Here's how the part is built. I have some questions about the finished solid (model axes, mm). Face numbers are marked on the shaded views. A direction names the side the tool comes from. Give positions to 0.01 mm unless a question says otherwise; leave off trailing zeros. Write each loop counter-clockwise with the first axis right and the second up, starting at its lowest first coordinate (ties: lowest second). Pieces come first, ordered by that corner, then holes. Notation, with made-up numbers: (42.5, 75) - (95.5, 75) arc R10 cw to (95.5, 88) - close; hole circle Ø2 at (88, -6.75). An arc over 180 degrees is marked (long way). One line per item, written item: value. Start each with the question number.
1) Imagine slicing it at D-D on x = 88. Write out the boundary of the cut face in (y, z), plus the area to 3 significant figures.
2) On a 3-axis mill with a long thin cutter (end or side, diameter ignored), from which of +Z, -Z, +X, -X, +Y, -Y can I reach the whole of each face in a straight line? I mean the marked faces 1 and 2. Say none if no direction works.
3) Imagine slicing it at A-A on x = 49.5. Write out the boundary of the cut face in (y, z), plus the area to 3 significant figures.
4) Imagine slicing it at C-C on y = 43.5. Write out the boundary of the cut face in (x, z), plus the area to 3 significant figures.
5) Imagine slicing it at B-B on z = 32. Write out the boundary of the cut face in (x, y).
6) I'm going to push flat-ended pins straight in: P1, Ø1, axis at x = 88.5, y = 43.5, coming from the +Z side; P2, Ø1.1, axis at x = 97.5, z = 19.5, coming from the -Y side; P3, Ø1.1, axis at y = 0, z = 21, coming from the +X side. Where does each tip first touch, or does it pass through?
7) Please list where these lines run through material, in increasing order: L1, parallel to Y at x = 10, z = 11; L2, parallel to X at y = 35.5, z = 11; L3, parallel to Y at x = 79, z = 36. Write a range as [from, to].
8) We'd pull the mould along X, two halves only. Please class the marked faces 3, 4, 5 and 6: +X half, -X half, draft (parallel to the pull), parting line (faces both ways), or undercut.
from build123d import *

# Parameters (mm, degrees)
SKICA1_W                 = 102
SKICA1_H                 = 65
P_IDAT_VYSUNUT_M1_DEPTH  = 3
SKICA1_4_W               = 102
SKICA1_4_H               = 65
SKICA1_4_W_2             = 98
SKICA1_4_H_2             = 61
P_IDAT_VYSUNUT_M2_DEPTH  = 39
SKICA1_5_W               = 98
SKICA1_5_H               = 61
SKICA1_5_W_2             = 94
SKICA1_5_H_2             = 57
P_IDAT_VYSUNUT_M3_DEPTH  = 34
SKICA2_W                 = 3.73
SKICA2_H                 = 6.55
ODEBRAT_VYSUNUT_M1_DEPTH = 4
ZAOBLIT1_R               = 3
ZAOBLIT2_R               = 3
ODEBRAT_START            = -0.45
SKICA4_W                 = 5.4
SKICA4_H                 = 5.4
ODEBRAT_VYSUNUT_M2_DEPTH = 3.55
ZAOBLIT3_R               = 3


with BuildPart() as part:
    # Skica1 → Přidat vysunutím1 (new body)
    with BuildSketch(Plane.XY):
        with Locations((49, 30.5)):
            Rectangle(SKICA1_W, SKICA1_H)
    extrude(amount=P_IDAT_VYSUNUT_M1_DEPTH)

    # Skica1<4> → Přidat vysunutím2 (add)
    with BuildSketch(Plane.XY):
        with Locations((49, 30.5)):
            Rectangle(SKICA1_4_W, SKICA1_4_H)
        with Locations((49, 30.5)):
            Rectangle(SKICA1_4_W_2, SKICA1_4_H_2, mode=Mode.SUBTRACT)
    extrude(amount=P_IDAT_VYSUNUT_M2_DEPTH)

    # Skica1<5> → Přidat vysunutím3 (add)
    with BuildSketch(Plane.XY):
        with Locations((49, 30.5)):
            Rectangle(SKICA1_5_W, SKICA1_5_H)
        with Locations((49, 30.5)):
            Rectangle(SKICA1_5_W_2, SKICA1_5_H_2, mode=Mode.SUBTRACT)
    extrude(amount=P_IDAT_VYSUNUT_M3_DEPTH)

    # Skica2 → Odebrat vysunutím1 (cut)
    with BuildSketch(Plane(origin=(100, 0, 0), x_dir=(0, 0, -1), z_dir=(1, 0, 0))):
        with Locations((-19.5, 30.5)):
            Rectangle(SKICA2_W, SKICA2_H)
    extrude(amount=-ODEBRAT_VYSUNUT_M1_DEPTH, mode=Mode.SUBTRACT)

    # Zaoblit1
    zaoblit1_edges = [part.edges().sort_by_distance(p)[0] for p in [
        (-2, 30.5, 0),
        (49, -2, 0),
        (100, 30.5, 0),
        (49, 63, 0),
    ]]
    fillet(zaoblit1_edges, radius=ZAOBLIT1_R)

    # Zaoblit2
    # the kernel refuses this fillet: 3 mm, written as the material it takes off along each edge
    with BuildSketch(Plane(origin=(97, 60, 3), x_dir=(1, 0, 0), z_dir=(0, 1, 0))) as zaoblit2_piece_1_section:
        Polygon((0, 0), (ZAOBLIT2_R, 0), (ZAOBLIT2_R, ZAOBLIT2_R), (0, ZAOBLIT2_R), align=None)
    zaoblit2_piece_1 = extrude(amount=ZAOBLIT2_R, mode=Mode.PRIVATE)
    zaoblit2_piece_1 = zaoblit2_piece_1 - Plane(origin=(97, 60, 3), x_dir=(-0.7071067811865475, 0, 0.7071067811865475), z_dir=(0, 1, 0)) * Sphere(ZAOBLIT2_R, mode=Mode.PRIVATE)
    add(zaoblit2_piece_1, mode=Mode.SUBTRACT)
    with BuildSketch(Plane(origin=(97, 1, 3), x_dir=(0, -1, 0), z_dir=(1, 0, 0))) as zaoblit2_piece_2_section:
        Polygon((0, 0), (ZAOBLIT2_R, 0), (ZAOBLIT2_R, ZAOBLIT2_R), (0, ZAOBLIT2_R), align=None)
    zaoblit2_piece_2 = extrude(amount=ZAOBLIT2_R, mode=Mode.PRIVATE)
    zaoblit2_piece_2 = zaoblit2_piece_2 - Plane(origin=(97, 1, 3), x_dir=(0, 0.7071067811865475, 0.7071067811865475), z_dir=(1, 0, 0)) * Sphere(ZAOBLIT2_R, mode=Mode.PRIVATE)
    add(zaoblit2_piece_2, mode=Mode.SUBTRACT)
    with BuildSketch(Plane(origin=(1, 60, 3), x_dir=(-1, 0, 0), z_dir=(0, 1, 0))) as zaoblit2_piece_3_section:
        Polygon((0, 0), (ZAOBLIT2_R, 0), (ZAOBLIT2_R, -ZAOBLIT2_R), (0, -ZAOBLIT2_R), align=None)
    zaoblit2_piece_3 = extrude(amount=ZAOBLIT2_R, mode=Mode.PRIVATE)
    zaoblit2_piece_3 = zaoblit2_piece_3 - Plane(origin=(1, 60, 3), x_dir=(0.7071067811865475, 0, 0.7071067811865475), z_dir=(0, 1, 0)) * Sphere(ZAOBLIT2_R, mode=Mode.PRIVATE)
    add(zaoblit2_piece_3, mode=Mode.SUBTRACT)
    with BuildSketch(Plane(origin=(1, 1, 3), x_dir=(0, -1, 0), z_dir=(-1, 0, 0))) as zaoblit2_piece_4_section:
        Polygon((0, 0), (ZAOBLIT2_R, 0), (ZAOBLIT2_R, -ZAOBLIT2_R), (0, -ZAOBLIT2_R), align=None)
    zaoblit2_piece_4 = extrude(amount=ZAOBLIT2_R, mode=Mode.PRIVATE)
    zaoblit2_piece_4 = zaoblit2_piece_4 - Plane(origin=(1, 1, 3), x_dir=(0, 0.7071067811865475, 0.7071067811865475), z_dir=(-1, 0, 0)) * Sphere(ZAOBLIT2_R, mode=Mode.PRIVATE)
    add(zaoblit2_piece_4, mode=Mode.SUBTRACT)
    with BuildSketch(Plane(origin=(-2, 63, 3), x_dir=(1, 0, 0), z_dir=(0, 0, 1)), Plane(origin=(-2, -2, 3), x_dir=(0, 1, 0), z_dir=(0, 0, 1)), Plane(origin=(100, -2, 46.5), x_dir=(0, 1, 0), z_dir=(0, 0, -1)), Plane(origin=(100, 63, 46.5), x_dir=(-1, 0, 0), z_dir=(0, 0, -1))) as zaoblit2_piece_5:
        with BuildLine():
            CenterArc((ZAOBLIT2_R, -ZAOBLIT2_R), ZAOBLIT2_R, 90, 90)
            Line((0, -ZAOBLIT2_R), (0, 0))
            Line((0, 0), (ZAOBLIT2_R, 0))
        make_face()
    extrude(amount=43.5, mode=Mode.SUBTRACT)

    # Skica4 → Odebrat vysunutím2 (cut)
    with BuildSketch(Plane.XZ.offset(2).offset(ODEBRAT_START)):
        with Locations((16.1, 21)):
            Rectangle(SKICA4_W, SKICA4_H)
        with Locations((32.55, 21)):
            Rectangle(SKICA4_W, SKICA4_H)
        with Locations((49, 21)):
            Rectangle(SKICA4_W, SKICA4_H)
        with Locations((65.45, 21)):
            Rectangle(SKICA4_W, SKICA4_H)
        with Locations((81.9, 21)):
            Rectangle(SKICA4_W, SKICA4_H)
    extrude(amount=-ODEBRAT_VYSUNUT_M2_DEPTH, mode=Mode.SUBTRACT)

    # Zaoblit3
    zaoblit3_edges = [part.edges().sort_by_distance(p)[0] for p in [
        (98, 61, 36.5),
        (98, 0, 36.5),
        (0, 0, 36.5),
        (0, 61, 36.5),
    ]]
    fillet(zaoblit3_edges, radius=ZAOBLIT3_R)


solid = part.part
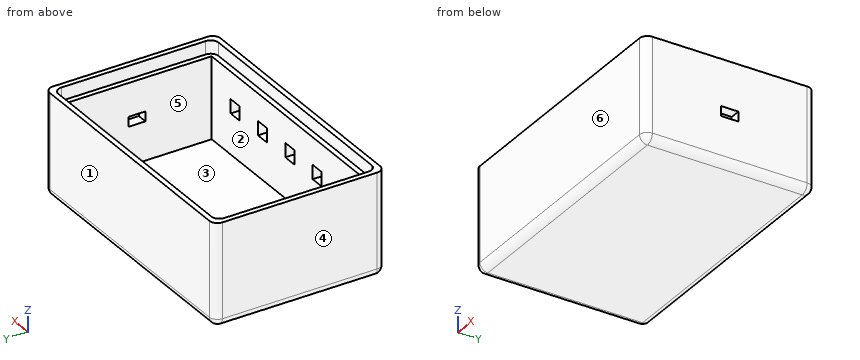
Numbers:
1. outline: (-2, 3) arc R3 ccw to (1, 0) - (60, 0) arc R3 ccw to (63, 3) - (63, 39) - (61, 39) - (61, 34) - (59, 34) - (59, 3) - (2, 3) - (2, 34) - (0, 34) - (0, 39) - (-2, 39) - close
1. area: 459 mm^2
2. face 1: +Z, -Z, +X, -X, +Y
2. face 2: +Z
3. outline: (-2, 3) arc R3 ccw to (1, 0) - (60, 0) arc R3 ccw to (63, 3) - (63, 39) - (61, 39) - (61, 34) - (59, 34) - (59, 3) - (2, 3) - (2, 18.3) - (-1.55, 18.3) - (-1.55, 23.7) - (2, 23.7) - (2, 34) - (0, 34) - (0, 39) - (-2, 39) - close
3. area: 440 mm^2
4. outline: (-2, 3) arc R3 ccw to (1, 0) - (97, 0) arc R3 ccw to (100, 3) - (100, 39) - (98, 39) - (98, 34) - (96, 34) - (96, 3) - (2, 3) - (2, 34) - (0, 34) - (0, 39) - (-2, 39) - close
4. area: 570 mm^2
5. outline: (-2, 1) arc R3 ccw to (1, -2) - (97, -2) arc R3 ccw to (100, 1) - (100, 60) arc R3 ccw to (97, 63) - (1, 63) arc R3 ccw to (-2, 60) - close; hole (2, 2) - (96, 2) - (96, 59) - (2, 59) - close
6. P1: z = 3
6. P2: y = -2
6. P3: x = 99.97
7. L1: [-2, 2], [59, 63]
7. L2: [-2, 2], [96, 100]
7. L3: [-2, 0], [61, 63]
8. face 3: undercut
8. face 4: -X half
8. face 5: undercut
8. face 6: draft
